Autodesk Inventor part; units mm, degrees
ref_plane "YZ Plane" through (0, 0, 0) normal (1, 0, 0) x (0, 1, 0)
ref_plane "XZ Plane" through (0, 0, 0) normal (0, 1, 0) x (-1, 0, 0)
ref_plane "XY Plane" through (0, 0, 0) normal (0, 0, 1) x (1, 0, 0)
sketch "Sketch1" plane through (0, 0, 0) normal (0, 0, 1) x (1, 0, 0)
  line L0 (-113.263, 0) -> (-213.263, 0)
  line L1 (-213.263, 0) -> (-213.263, 300)
  line L2 (-213.263, 300) -> (-113.263, 300)
  line L3 (-113.263, 300) -> (-113.263, 0)
  circle A0 centre (-163.263, 32) radius 6
  circle A1 centre (-191.263, 278) radius 6
  circle A2 centre (-135.263, 278) radius 6
  point P0 (0, 0)
  dimension "d0" = 100
  dimension "d1" = 300
  dimension "d2" = 12
  dimension "d3" = 32
  dimension "d4" = 12
  dimension "d5" = 22
  dimension "d6" = 22
  dimension "d7" = 12
  dimension "d8" = 22
  dimension "d9" = 22
extrude "Extrusion1" add sketch "Sketch1" along normal blind 44
sketch "Sketch2" plane through (0, 0, 44) normal (0, 0, 1) x (1, 0, 0)
  line L0 (-113.263, 300) -> (-213.263, 300)
  line L1 (-213.263, 300) -> (-213.263, 280)
  line L2 (-213.263, 300) -> (-213.263, 0)
  line L3 (-213.263, 280) -> (-113.263, 280)
  line L4 (-113.263, 0) -> (-113.263, 300)
  line L5 (-113.263, 280) -> (-113.263, 300)
  line L6 (-213.263, 300) -> (-113.263, 300)
  line L7 (-213.263, 0) -> (-213.263, 20)
  line L8 (-213.263, 0) -> (-113.263, 0)
  line L9 (-213.263, 0) -> (-113.263, 0)
  line L10 (-113.263, 0) -> (-113.263, 20)
  line L11 (-213.263, 20) -> (-113.263, 20)
  line L12 (-113.263, 20) -> (-113.263, 280)
  line L13 (-213.263, 20) -> (-213.263, 280)
  point P0 (0, 0)
  dimension "d12" = 20
  dimension "d13" = 20
extrude "Extrusion2" cut sketch "Sketch2" against normal blind 24 contours L4 L11 L2 L3
ref_plane "Work Plane1" through (-163.263, 0, 0) normal (-1, 0, 0) x (0, 0, 1)
sketch "Sketch6" plane through (-163.263, 0, 0) normal (-1, 0, 0) x (0, 0, 1)
  line L0 (44, 284) -> (44, 280)
  circle A0 centre (-256, 280) radius 26
  point P0 (0, 0)
  dimension "d24" = 52
extrude "Extrusion5" add sketch "Sketch6" along normal mid plane 76
sketch "Sketch7" plane through (-201.263, 280, -256) normal (-1, 0, 0) x (0, 0, 1)
  circle A0 centre (0, 0) radius 20
  point P0 (256, -280)
  dimension "d27" = 40
extrude "Extrusion6" cut sketch "Sketch7" against normal blind 76
sketch "Sketch9" plane through (-163.263, 0, 0) normal (-1, 0, 0) x (0, 0, 1)
  line L0 (44, 284) -> (44, 280)
  circle A0 centre (-256, 280) radius 26
  line L1 (0, 300) -> (0, 0)
  circle A1 centre (-256, 280) radius 26
  line L2 (0, 230) -> (-228, 230)
  line L3 (-230, 232) -> (-230, 280)
  line L4 (0, 230) -> (0, 218)
  line L5 (0, 218) -> (-240, 218)
  line L6 (-242, 220) -> (-242, 253)
  arc A2 (-230, 232) -> (-228, 230) centre (-228, 232) ccw
  arc A3 (-242, 220) -> (-240, 218) centre (-240, 220) ccw
  line L7 (-242, 253) -> (-250.7822, 253) construction
  line L8 (-243.1836, 257.3871) -> (-250.7822, 253) construction
  arc A4 (-242, 253) -> (-243.1836, 257.3871) centre (-250.7225, 253) ccw
  point P0 (-242, 218)
  point P1 (-243.1797, 257.3805)
  dimension "d35" = 52
  dimension "d37" = 12
  dimension "d38" = 242
  dimension "d39" = 35
  dimension "d40" = 2
  dimension "d41" = 2
  dimension "d42" = 30
extrude "Extrusion7" add sketch "Sketch9" along normal blind 50 contours L3 A2 L2 L1 L5 A3 L6 A4 A0
sketch "Sketch10" plane through (-163.263, 230, 0) normal (0, 1, 0) x (1, 0, 0)
  line L0 (-50, 0) -> (-41.2717, 264.4302)
  line L1 (-41.2717, 264.4302) -> (-54.1734, 264.856)
  line L2 (-54.1734, 264.856) -> (-50, 0)
  point P0 (163.263, 0)
extrude "Extrusion8" cut sketch "Sketch10" against normal blind 50
sketch "Sketch12" plane through (-213.263, 232, -230) normal (-1, 0, 0) x (0, 0, 1)
  line L0 (-12, 21) -> (-12, -2)
  line L1 (0, 48) -> (2.6747, 48)
  line L2 (-12, 48) -> (0, 48)
  line L3 (2.6747, 48) -> (2.6747, -2)
  line L4 (2, -2) -> (230, -2)
  line L5 (-12, -2) -> (2.6747, -2)
  line L6 (-12, -2) -> (-15.3342, -2)
  line L7 (-15.3342, -2) -> (-15.3342, 48)
  line L8 (-15.3342, 48) -> (-11.4757, 48)
  point P0 (230, -232)
extrude "Extrusion9" cut sketch "Sketch12" against normal blind 12
sketch "Sketch13" plane through (-163.263, 230, 0) normal (0, 1, 0) x (1, 0, 0)
  line L0 (-38, 228) -> (-38, 242)
  line L1 (-38, 228) -> (-50, 0)
  line L2 (-42.012, 242) -> (-38, 242)
  line L3 (-50, 0) -> (-42.012, 242)
  line L4 (-42.012, 242) -> (-38, 242)
  line L5 (-38, 242) -> (-38, 228)
  point P0 (163.263, 0)
extrude "Extrusion10" cut sketch "Sketch13" against normal blind 12
properties part number "6 - Part 6"
Could you check a few things on this model? Use its own coordinates, in mm. A direction names the side the tool comes from. Round coordinates to 2 decimals unless told otherwise and drop trailing zeros. Loops run counter-clockwise (first coordinate to the right, second up) from the corner with the lowest first, then second, coordinate; pieces in that order, holes last. Notation, with made-up numbers: (67, 67.5) - (89, 67.5) arc R15 ccw to (89, 94.5) - close; hole circle Ø3 at (-21, 55.5). An arc over 180 degrees is marked (long way). Use CSV: the item, a comma, the result in double quotes.
Item 1: If we section it at B-B on y = 245: List the corners of the cut face in (x, z) for me.
Here are the results:
outline,"(-213.26, 0) - (-113.26, 0) - (-113.26, 20) - (-213.26, 20) - close; (-201.26, -242) - (-163.26, -242) - (-163.26, -230) - (-201.26, -230) - close"
Item 2: If we section it at C-C on z = 16: List the corners of the cut face in (x, y) for me, then the cut area to 3 significant figures.
Here are the results:
outline,"(-213.26, 0) - (-113.26, 0) - (-113.26, 300) - (-213.26, 300) - close; hole circle Ø12 at (-191.26, 278); hole circle Ø12 at (-163.26, 32); hole circle Ø12 at (-135.26, 278)"
area,"29,700 mm²"
Item 3: If we mould it in two halves opening along Y, with no side actions, what happens to faces 1 (the flat face through (-163, 0, 22)), 2 (the cylindrical face through (-157.72, 34.3, 9.86)), 3 (the flat face through (-182, 256, -230)), 4 (the flat face through (-164, 152, 20))? For each: pulls with the +Y half, pulls with the -Y half, needs draft (parallel to the pull), parting line crosses it, or undercut.
Here are the results:
face 1,"pulls with the -Y half"
face 2,"undercut"
face 3,"needs draft"
face 4,"undercut"
Item 4: If we section it at A-A on x = -146: List the corners of the cut face in (y, z) for me.
Here are the results:
outline,"(0, 0) - (300, 0) - (300, 44) - (280, 44) - (280, 20) - (20, 20) - (20, 44) - (0, 44) - close; circle Ø52 at (280, -256); hole circle Ø40 at (280, -256)"
Item 5: If we section it at D-D on x = -175.5: List the corners of the cut face in (y, z) for me.
Here are the results:
outline,"(0, 0) - (218, 0) - (218, -240) arc R2 ccw to (220, -242) - (253, -242) arc R8.72 cw to (257.38, -243.18) arc R26 ccw (long way) to (280, -230) - (232, -230) arc R2 cw to (230, -228) - (230, 0) - (300, 0) - (300, 44) - (280, 44) - (280, 20) - (20, 20) - (20, 44) - (0, 44) - close; hole circle Ø40 at (280, -256)"
Item 6: Will these pins go through, and if not, where does the flat tip stop? pin 1 (13 mm diameter, centred on x = -201.5, z = 28, fed in from -Y); pin 2 (19 mm diameter, centred on x = -163.263, y = 32, fed in from -Z); pin 3 (18.5 mm diameter, centred on y = 236, z = -101, fed in from +X); pin 4 (11.5 mm diameter, centred on x = -179.5, y = 247.5, fed in from +Z).
Here are the results:
pin 1,"stops at y = 0"
pin 2,"stops at z = 0"
pin 3,"stops at x = -163.26"
pin 4,"stops at z = 20"
Item 7: I need wall thicknesses on L1, parallel to X at y = 278, z = 17; L2, parallel to Y at x = -181, z = -163; L3, parallel to X at y = 32, z = 13. Which ranges of each line are inside material? Lowest first, please. Write a range as [from, to].
Here are the results:
L1,"x = [-213.26, -197.26], [-185.26, -141.26], [-129.26, -113.26]"
L2,"y = [218, 230]"
L3,"x = [-213.26, -169.26], [-157.26, -113.26]"
Item 8: For faces 5 (the cylindrical face through (-136.56, 283.86, 16.8)), 6 (the flat face through (-125.263, 264.7, -242.6)), 7 (the cylindrical face through (-162.731, 295.821, -276.633)), 8 (the flat face through (-201.263, 262, -243)), which set-ups out of +Z, -Z, +X, -X, +Y, -Y let a thin tool reach every point of the face, with its end or its side?
Here are the results:
face 5,"+Z"
face 6,"-Z, +X, +Y, -Y"
face 7,"+X"
face 8,"-Z, -X, +Y, -Y"
